Autodesk Inventor part; units mm, degrees
ref_plane "YZ Plane" through (0, 0, 0) normal (1, 0, 0) x (0, 1, 0)
ref_plane "XZ Plane" through (0, 0, 0) normal (0, 1, 0) x (-1, 0, 0)
ref_plane "XY Plane" through (0, 0, 0) normal (0, 0, 1) x (1, 0, 0)
sketch "Sketch1" plane through (0, 0, 0) normal (0, 1, 0) x (-1, 0, 0)
  line L0 (0, 0) -> (0, -8)
  line L1 (0, 0) -> (-4.5, 0)
  arc A0 (-4.7918, -2) -> (-4.5, 0) centre (-11.5, 0) ccw
  line L2 (-6, -5.1202) -> (0, -5.1202)
  arc A1 (-6, -5.1202) -> (-4.7918, -2) centre (-14.5898, 0) ccw
  dimension "d6" = 8
  dimension "d7" = 7
  dimension "d9" = 12
  dimension "d10" = 9
  dimension "d11" = 10
  dimension "d12" = 2
revolve "Revolution1" add sketch "Sketch1" angle 360 about axis through (0, 0, 0) along (0, 0, -1)
sketch "Sketch2" plane through (0, 0, 0) normal (0, 0, 1) x (1, 0, 0)
  circle A0 centre (0, 0) radius 4.5 construction
hole "Hole1" at (0, 0, 0) direction (0, 0, -1) diameter 7 depth 5.1202
fillet "Fillet1" radius 1 1 edges at (-4.7918, 0, -2)
properties part number "VenturiEinsatz" material "Copper"
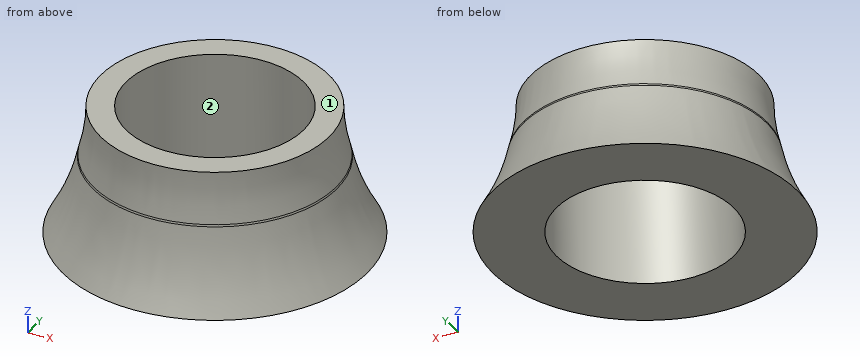
Design review of the part built by this model. Coordinates are the model's own, in mm. Face numbers are marked on the shaded views. Coordinates: 2 decimals unless noted, no trailing zeros. Order: outer loops, then holes, each group sorted by start corner. A loop starts at its lowest first (then second) coordinate and runs counter-clockwise, first axis right, second up. Notation, with made-up numbers: (61, -20) -> (67, -20) arc R18 cw to (67, -13) -> close; hole circle Ø4 at (84.5, -6). An arc over 180 degrees is marked (long way). One line per item, written item: value. Start each with the question number.
Q1. Take a section at C-C, the plane z = -0.3. State the section outline as (x, y) points, then the cut area to 3 significant figures.
Q2. Take a section at A-A, the plane y = 0. State the section outline as (x, z) points.
Q3. Mouldability with a two-part tool opening along Y and no side actions: class the marked faces 1 and 2 as pulls with the +Y half, pulls with the -Y half, needs draft (parallel to the pull), parting line crosses it, or undercut.
Q4. Take a section at B-B, the plane z = -1.8. State the section outline as (x, y) points, then the cut area to 3 significant figures.
Q5. For probe 1 along Y at (x, z) = (0, -1.95); probe 2 along Y at (x, z) = (-2, -1.1); probe 3 along X at (y, z) = (0, -3.25), list the stretches that pass through material, from the lowest coordinate up.
Q6. Insertion check: pin 1 Ø2 at (x, z) = (-2.5, -4) entering from -Y; pin 2 Ø3 at (y, z) = (-4.5, -3.5) entering from -X. Each pin has a flat end and moves straight along its axis. Give the tip position at first contact, or say it passes through.
Values follow:
1. outline: circle Ø9.01 at (0, 0); hole circle Ø7 at (0, 0)
1. area: 25.3 mm2
2. outline: (-6, -5.12) -> (-3.5, -5.12) -> (-3.5, 0) -> (-4.5, 0) arc R7 cw to (-4.78, -1.96) arc R1 ccw to (-4.8, -2.04) arc R10 cw to start; (3.5, -5.12) -> (6, -5.12) arc R10 cw to (4.8, -2.04) arc R1 ccw to (4.78, -1.96) arc R7 cw to (4.5, 0) -> (3.5, 0) -> close
3. face 1: needs draft
3. face 2: undercut
4. outline: circle Ø9.47 at (0, 0); hole circle Ø7 at (0, 0)
4. area: 32.0 mm2
5. probe 1: y = -4.78 to -3.5, 3.5 to 4.78
5. probe 2: y = -4.13 to -2.87, 2.87 to 4.13
5. probe 3: x = -5.13 to -3.5, 3.5 to 5.13
6. pin 1: stops at y = -5.5
6. pin 2: stops at x = -4.54
